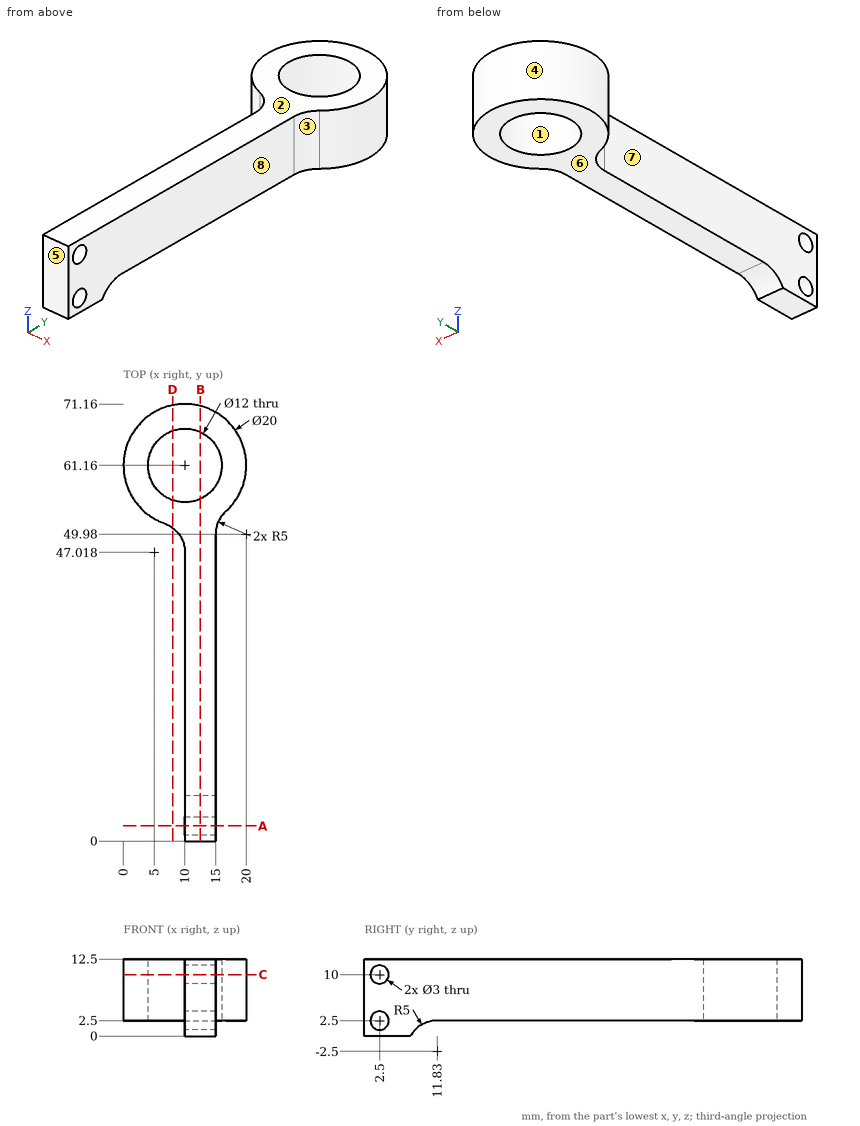
Verification items for this drawing (mm, ordinates from the low corner). A direction names the side the tool comes from. Coordinates: 2 decimals unless noted, no trailing zeros. Order: outer loops, then holes, each group sorted by start corner. A loop starts at its lowest first (then second) coordinate and runs counter-clockwise, first axis right, second up.
Q1. Sectioned sample at B-B on x = 12.5. Record the cut outline in (y, z) (1 decimal), and give its area (3 significant figures).
Reply:
outline: (0, 0) - (7.5, 0) arc R5 cw to (11.8, 2.5) - (55.7, 2.5) - (55.7, 12.5) - (0, 12.5) - close; (66.6, 2.5) - (70.8, 2.5) - (70.8, 12.5) - (66.6, 12.5) - close; hole circle Ø3 at (2.5, 2.5); hole circle Ø3 at (2.5, 10)
area: 607 mm2
Q2. Depth check by flat-ended pin: pin 1 Ø6 at (y, z) = (24, 5.5) entering from +X; pin 2 Ø8 at (x, y) = (6.5, 34.5) entering from -Z. Enter the tip coordinate at first touch or a pass-through.
Reply:
pin 1: stops at x = 15
pin 2: stops at z = 2.5
Q3. Sectioned sample at A-A on y = 2.5. Record the cut outline in (x, z), and give its area (3 significant figures).
Reply:
outline: (10, 0) - (15, 0) - (15, 1) - (10, 1) - close; (10, 4) - (15, 4) - (15, 8.5) - (10, 8.5) - close; (10, 11.5) - (15, 11.5) - (15, 12.5) - (10, 12.5) - close
area: 32.5 mm2
Q4. Tool access check on the marked faces 4, 5, 6, 7 and 8. Record the directions out of +Z, -Z, +X, -X, +Y, -Y that give a thin tool (end or side, any length) a straight path to the whole face; none if there is none.
Reply:
face 4: +Z, -Z
face 5: +Z, -Z, +X, -X, -Y
face 6: -Z, +X, -X, +Y
face 7: +Z, -Z, -X, -Y
face 8: +Z, -Z, +X, -Y
Q5. Sectioned sample at C-C on z = 10. Record the cut outline in (x, y).
Reply:
outline: (6.67, 51.73) arc R5 cw to (10, 47.02) - (10, 4) - (15, 4) - (15, 49.98) arc R5 cw to (16.67, 53.71) arc R10 ccw (long way) to start; (10, 0) - (15, 0) - (15, 1) - (10, 1) - close; hole circle Ø12 at (10, 61.16)
Q6. Draft check along Y on the marked faces 1, 2 and 3. Enter one of: released by +Y, released by -Y, zero draft, split by the parting line, or undercut.
Reply:
face 1: undercut
face 2: zero draft
face 3: released by -Y
Q7. Thickness scan on probe 1 along Z at (x, y) = (11.35, 2.5); probe 2 along Z at (x, y) = (12.5, 12); probe 3 along X at (y, z) = (22, 7). Record the ranges inside material, lowest first.
Reply:
probe 1: z = 0 to 1, 4 to 8.5, 11.5 to 12.5
probe 2: z = 2.5 to 12.5
probe 3: x = 10 to 15
Q8. Sectioned sample at D-D on x = 8. Record the cut outline in (y, z).
Reply:
outline: (51.02, 2.5) - (55.5, 2.5) - (55.5, 12.5) - (51.02, 12.5) - close; (66.82, 2.5) - (70.96, 2.5) - (70.96, 12.5) - (66.82, 12.5) - close
